Can you work these out from the drawing? Everything is in mm from the part's minimum corner. A direction names the side the tool comes from. Coordinates: 2 decimals unless noted, no trailing zeros. Order: outer loops, then holes, each group sorted by start corner. A loop starts at its lowest first (then second) coordinate and runs counter-clockwise, first axis right, second up. Notation, with made-up numbers: (73, 85) -> (111, 85) arc R7 cw to (111, 92) -> close; hole circle Ø3 at (51.25, 13.5). An arc over 180 degrees is marked (long way). Return JSON: item names as keys, results as strings. Group by question number.
1) If we section it at A-A, the plane x = 21: Please give me the cut outline in (y, z), then the cut area to 3 significant figures.
2) If we section it at C-C, the plane y = 54.5: Please give me the cut outline in (x, z), then the cut area to 3 significant figures.
3) Thinking about a two-plate mould opening in X: for the marked faces 1, 2, 3 and 4, which applies, +X half, -X half, draft (parallel to the pull), parting line (faces both ways), or undercut?
4) If we section it at D-D, the plane z = 13: Please give me the cut outline in (x, y), then the cut area to 3 significant figures.
5) For pin 1 (10 mm diameter, centred on x = 35.5, z = 37.5, fed in from +Y); pin 2 (12 mm diameter, centred on x = 8.5, y = 64.5, fed in from +Z), each with a flat end and sliding along its axis, tell me the tip position at first contact or that it passes through.
6) If I drill on probe 1 along Y at (x, z) = (17, 12.5); probe 2 along Y at (x, z) = (31, 6), over which ranges is the centre line in solid material (lowest first)? Write a range as from..to.
7) For the marked faces 5 and 6, which set-ups out of +Z, -Z, +X, -X, +Y, -Y let a thin tool reach every point of the face, with its end or its side?
8) If we section it at B-B, the plane z = 21: Please give me the cut outline in (x, y), then the cut area to 3 significant figures.
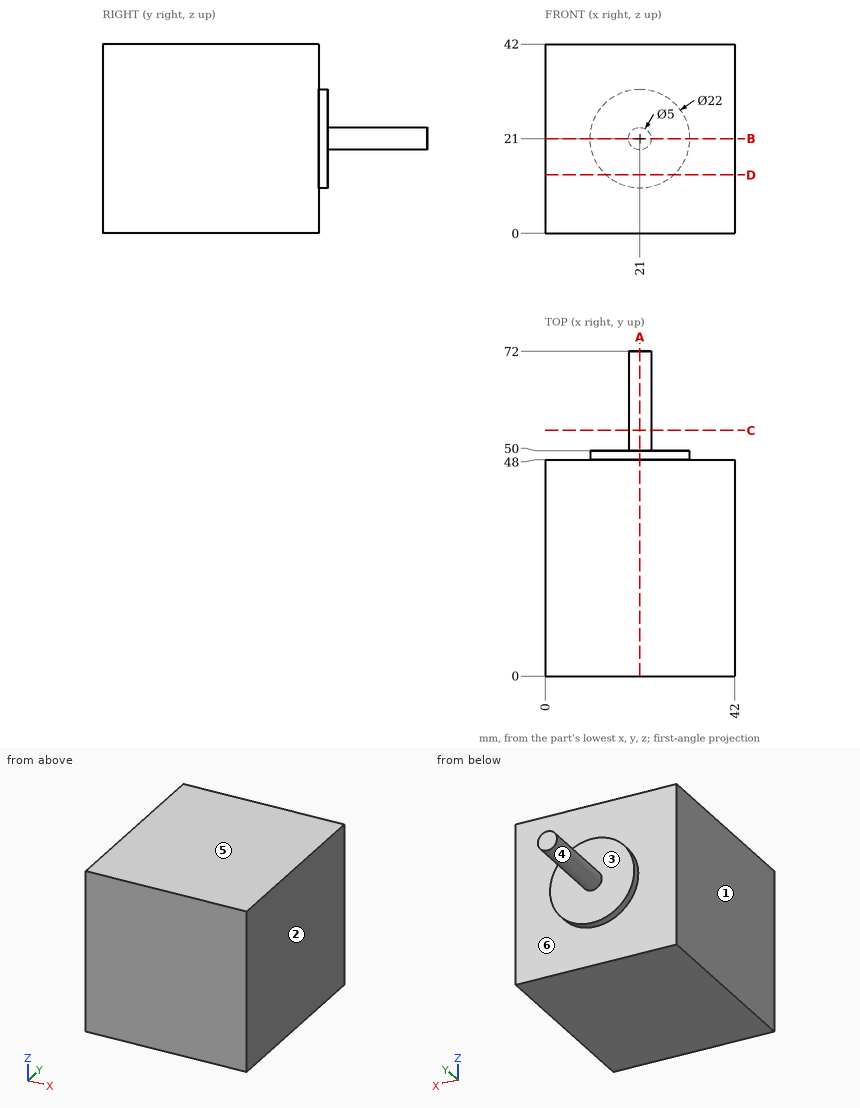
Result sheet:
{
 "1": {"outline": "(0, 0) -> (48, 0) -> (48, 10) -> (50, 10) -> (50, 18.5) -> (72, 18.5) -> (72, 23.5) -> (50, 23.5) -> (50, 32) -> (48, 32) -> (48, 42) -> (0, 42) -> close", "area": "2,170 mm2"},
 "2": {"outline": "circle Ø5 at (21, 21)", "area": "19.6 mm2"},
 "3": {"face 1": "-X half", "face 2": "+X half", "face 3": "draft", "face 4": "parting line"},
 "4": {"outline": "(0, 0) -> (42, 0) -> (42, 48) -> (28.55, 48) -> (28.55, 50) -> (13.45, 50) -> (13.45, 48) -> (0, 48) -> close", "area": "2,050 mm2"},
 "5": {"pin 1": "stops at y = 48", "pin 2": "passes through"},
 "6": {"probe 1": "y = 0..50", "probe 2": "y = 0..48"},
 "7": {"face 5": "+Z, +X, -X, +Y, -Y", "face 6": "+Y"},
 "8": {"outline": "(0, 0) -> (42, 0) -> (42, 48) -> (32, 48) -> (32, 50) -> (23.5, 50) -> (23.5, 72) -> (18.5, 72) -> (18.5, 50) -> (10, 50) -> (10, 48) -> (0, 48) -> close", "area": "2,170 mm2"}
}
